```python
from build123d import *

# Parameters (mm, degrees)
EXTRUDE_1_DEPTH          = 6
PATTERN_CIRCULAR_1_COUNT = 6
FILLET_1_R               = 3


with BuildPart() as part:
    # 草图1 → 凸台-拉伸1 (new body)
    with BuildSketch(Plane(origin=(0, 0, 0), x_dir=(1, 0, 0), z_dir=(0, 1, 0))):
        with BuildLine():
            Line((-3, 15.716233646), (-3, 25.716233646))
            ThreePointArc((-3, 25.716233646), (0.201439561, 33.447280184), (7.931262854, 36.651672125))
            Line((7.931262854, 36.651672125), (7.931262854, 30.651671155))
            ThreePointArc((7.931262854, 30.651671155), (4.44408042, 29.204639325), (3, 25.716233646))
            Line((3, 25.716233646), (3, 15.716233646))
            ThreePointArc((3, 15.716233646), (8, 13.856406461), (12.110657589, 10.456193034))
            Line((12.110657589, 10.456193034), (3.027664397, 2.614048259))
            Line((3.027664397, 2.614048259), (-0.75, 3.929058411))
            Line((-0.75, 3.929058411), (-3, 15.716233646))
        make_face()
    extrude_1 = extrude(amount=EXTRUDE_1_DEPTH)

    # 阵列(圆周)1: 凸台-拉伸1 ×6 about axis
    pattern_circular_1_axis = Axis((0, 0, 0), (0, 1, 0))
    for i in range(1, PATTERN_CIRCULAR_1_COUNT):
        add(extrude_1.rotate(pattern_circular_1_axis, i * 360 / PATTERN_CIRCULAR_1_COUNT))

    # 圆角1
    fillet_1_edges = [part.edges().sort_by_distance(p)[0] for p in [
        (-3, 3, -15.716233646),
        (3, 3, -15.716233646),
        (12.110657589, 3, -10.456193034),
        (-12.110657589, 3, -10.456193034),
        (-15.110657589, 3, -5.260040611),
        (-15.110657589, 3, 5.260040611),
        (-12.110657589, 3, 10.456193034),
        (-3, 3, 15.716233646),
        (3, 3, 15.716233646),
        (12.110657589, 3, 10.456193034),
        (15.110657589, 3, 5.260040611),
        (15.110657589, 3, -5.260040611),
    ]]
    fillet(fillet_1_edges, radius=FILLET_1_R)


solid = part.part
```
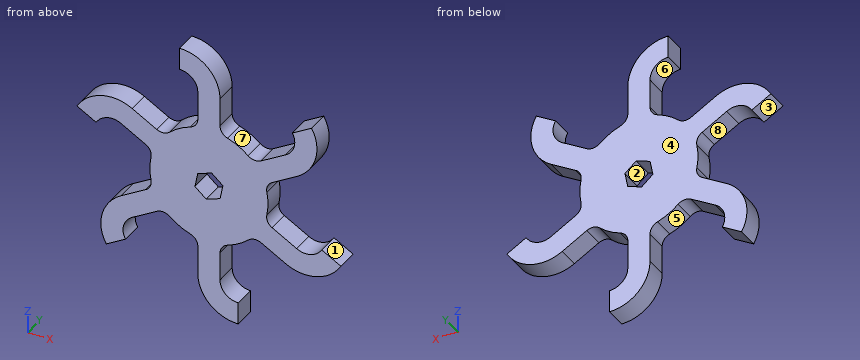
Verification items for the finished model (mm, model axes). Face numbers are marked on the shaded views. A direction names the side the tool comes from. Coordinates: 2 decimals unless noted, no trailing zeros. Loops run counter-clockwise (first coordinate to the right, second up) from the corner with the lowest first, then second, coordinate; pieces in that order, holes last. Notation, with made-up numbers: (14.25, 51.5) -> (38.25, 51.5) arc R27 ccw to (38.25, 84.5) -> close; hole circle Ø3 at (-27.5, -16). An arc over 180 degrees is marked (long way). Answer in a Markdown table with one row per item.
1) Scan lines: line 1 along X through (y, z) = (0.2, 20); line 2 along X through (y, z) = (3.2, 4); line 3 along Z through (x, y) = (17, 4.95). Record each from-to range of solid material in increasing order. Write a range as from..to.
The answers:
| item | result |
|---|---|
| line 1 | x = -3..3, 23.23..29.24 |
| line 2 | x = -15.62..15.62 |
| line 3 | z = -13.28..-6.35, 6.35..13.28 |
2) Section check B-B (z = 28). Record the cut outline in (x, y).
The answers:
| item | result |
|---|---|
| outline | (-3.56, 0) -> (2.76, 0) -> (2.76, 6) -> (-3.56, 6) -> close |
3) Section check D-D (z = 5). Record the cut outline in (x, y).
The answers:
| item | result |
|---|---|
| outline | (-15.86, 0) -> (15.86, 0) -> (15.86, 6) -> (-15.86, 6) -> close |
4) Depth check by flat-ended pin: P1, Ø3, axis at y = 4, z = -34, coming from the +X side; P2, Ø1, axis at y = 4, z = 13.5, coming from the +X side; P3, Ø3, axis at y = 3.5, z = 23.5, coming from the -X side; P4, Ø5, axis at x = -16.5, z = 17.5, coming from the +Y side. Enter the tip coordinate at first touch or a pass-through.
The answers:
| item | result |
|---|---|
| P1 | stops at x = 7.93 |
| P2 | stops at x = 27.62 |
| P3 | stops at x = -3 |
| P4 | passes through |
5) Section check C-C (x = -6). Record the cut outline in (y, z), and give its area (3 significant figures).
The answers:
| item | result |
|---|---|
| outline | (0, -14.83) -> (6, -14.83) -> (6, 14.83) -> (0, 14.83) -> close; (0, 30.26) -> (6, 30.26) -> (6, 36.48) -> (0, 36.48) -> close |
| area | 215 mm2 |
6) Access from +Z, -Z, +X, -X, +Y, -Y to the whole of each face (thin tool, end or side, straight path). Record for the marked faces 5, 6, 7 and 8.
The answers:
| item | result |
|---|---|
| face 5 | -Z, +Y, -Y |
| face 6 | -X, +Y, -Y |
| face 7 | +Z, +Y, -Y |
| face 8 | +Y, -Y |
7) Section check A-A (x = 19). Record the cut outline in (y, z), and give its area (3 significant figures).
The answers:
| item | result |
|---|---|
| outline | (0, -14.43) -> (6, -14.43) -> (6, -7.51) -> (0, -7.51) -> close; (0, 7.51) -> (6, 7.51) -> (6, 14.43) -> (0, 14.43) -> close |
| area | 83.1 mm2 |
8) Draft check along X on the marked faces 1, 2, 3 and 4. Enter one of: released by +X, released by -X, zero draft, split by the parting line, or undercut.
The answers:
| item | result |
|---|---|
| face 1 | released by +X |
| face 2 | undercut |
| face 3 | released by -X |
| face 4 | zero draft |
